```python
from build123d import *

# Parameters (mm, degrees)
SKETCH2_R          = 3.175
CUT_EXTRUDE1_DEPTH = 224.79
CIRPATTERN1_COUNT  = 8


with BuildPart() as part:
    # Sketch1 → Revolve1 (revolve)
    with BuildSketch(Plane.XY):
        Polygon((0, 76.2), (127.635, 76.2), (127.635, 89.7128), (126.8222, 89.7128), (126.8222, 77.0128), (0.8128, 77.0128), (0.8128, 89.7128), (0, 89.7128), align=None)
    revolve(axis=Axis((0, 0, 0), (1, 0, 0)))

    # Sketch2 → Cut-Extrude1 (cut)
    with BuildSketch(Plane(origin=(0, 0, 0), x_dir=(0, 0, -1), z_dir=(1, 0, 0))):
        with Locations((0, 85.09)):
            Circle(SKETCH2_R)
    cut_extrude1 = extrude(amount=CUT_EXTRUDE1_DEPTH, mode=Mode.SUBTRACT)

    # CirPattern1: Cut-Extrude1 ×8 about axis
    cirpattern1_axis = Axis((0, 0, 0), (1, 0, 0))
    for i in range(1, CIRPATTERN1_COUNT):
        add(cut_extrude1.rotate(cirpattern1_axis, i * 360 / CIRPATTERN1_COUNT), mode=Mode.SUBTRACT)


solid = part.part
```
Design review of the part built by this model. Coordinates are the model's own, in mm. Give positions to 0.01 mm unless a question says otherwise; leave off trailing zeros. Order: outer loops, then holes, each group sorted by start corner. A loop starts at its lowest first (then second) coordinate and runs counter-clockwise, first axis right, second up. Notation, with made-up numbers: (35.5, 49) - (43.5, 49) arc R36 ccw to (43.5, 84) - close; hole circle Ø9 at (-23.5, -40). An arc over 180 degrees is marked (long way). Use a Markdown table: item, result. Add a question column.
(1) Add section A-A on y = -85.09. Give the boundary of the cut face in (x, z) (3 decimals).
(2) Wall thickness on probe 1 along X at (y, z) = (-58.5, -56.5) (3 decimals); probe 2 along Z at (x, y) = (27.5, 15); probe 3 along Z at (x, y) = (95, 40): over which ranges is each line inside the solid? List them lowest first. Write a range as [from, to].
(3) Add section C-C on z = 0. Give the number of separate pieces and of enclosed holes in the cut face, then the cut area to 3 significant figures.
(4) Clearance check with flat-ended pins moving along their axes: P1, Ø1.5, axis at x = 82.5, z = 25, coming from the -Y side; P2, Ø6, axis at x = 66, z = -31, coming from the -Y side; P3, Ø10, axis at x = 19, y = -42.5, coming from the -Z side. State where each tip first meets the part, or that it passes through.
(5) Add section D-D on x = 71. Give the boundary of the cut face in (y, z).
(6) Mouldability with a two-part tool opening along X and no side actions: class faces 1 (the face through (127.635, 20, 74)), 2 (the face through (127.22, 0.41, -88.24)), 3 (the face through (0.813, 0, -79)) as +X half, -X half, draft (parallel to the pull), parting line (faces both ways), or undercut.
Report:
| question | item | result |
|---|---|---|
| 1 | outline | (0, -28.427) - (0.813, -28.427) - (0.813, -3.175) - (0, -3.175) - close; (0, 3.175) - (0.813, 3.175) - (0.813, 28.427) - (0, 28.427) - close; (126.822, -28.427) - (127.635, -28.427) - (127.635, -3.175) - (126.822, -3.175) - close; (126.822, 3.175) - (127.635, 3.175) - (127.635, 28.427) - (126.822, 28.427) - close |
| 2 | probe 1 | x = [0, 0.813], [126.822, 127.635] |
| 2 | probe 2 | z = [-75.54, -74.71], [74.71, 75.54] |
| 2 | probe 3 | z = [-65.81, -64.86], [64.86, 65.81] |
| 3 | separate pieces | 6 |
| 3 | enclosed holes | 0 |
| 3 | area | 228 mm² |
| 4 | P1 | stops at y = -73.1 |
| 4 | P2 | stops at y = -71.74 |
| 4 | P3 | stops at z = -67.27 |
| 5 | outline | circle Ø154.03 at (0, 0); hole circle Ø152.4 at (0, 0) |
| 6 | face 1 | +X half |
| 6 | face 2 | draft |
| 6 | face 3 | undercut |
